```python
from build123d import *

# Parameters (mm, degrees)
SKETCH_1_R          = 4.5
EXTRUDE_1_DEPTH     = 2
SKETCH_2_R          = 3.5
CUT_EXTRUDE_1_DEPTH = 2
SKETCH_3_R          = 1.5
CUT_EXTRUDE_2_DEPTH = 7.670832032


with BuildPart() as part:
    # 草图1 → 凸台-拉伸1 (new, symmetric)
    with BuildSketch(Plane(origin=(0, 0, 0), x_dir=(1, 0, 0), z_dir=(0, 1, 0))):
        with Locations(Location((0, 0, 0), (0, 0, 270))):
            Circle(SKETCH_1_R)
    extrude(amount=EXTRUDE_1_DEPTH, both=True)

    # 草图2 → 切除-拉伸1 (cut)
    with BuildSketch(Plane(origin=(0, 2, 0), x_dir=(1, 0, 0), z_dir=(0, 1, 0))):
        with Locations(Location((0, 0, 0), (0, 0, 270))):
            Circle(SKETCH_2_R)
    extrude(amount=-CUT_EXTRUDE_1_DEPTH, mode=Mode.SUBTRACT)

    # 草图3 → 切除-拉伸2 (cut, through all)
    with BuildSketch(Plane(origin=(0, 0, 0), x_dir=(1, 0, 0), z_dir=(0, 1, 0))):
        with Locations(Location((0, 0, 0), (0, 0, 270))):
            Circle(SKETCH_3_R)
    extrude(amount=-CUT_EXTRUDE_2_DEPTH, mode=Mode.SUBTRACT)


solid = part.part
```
Work out the finished part from the listing and answer in its coordinate system (mm). Coordinates: 2 decimals unless noted, no trailing zeros. Loops run counter-clockwise (first coordinate to the right, second up) from the corner with the lowest first, then second, coordinate; pieces in that order, holes last. Notation, with made-up numbers: (1.25, 35.25) - (22.25, 35.25) arc R29 cw to (22.25, 70.25) - close; hole circle Ø3 at (44.5, 75). An arc over 180 degrees is marked (long way). Use a Markdown table: item, result.
Item 1: Find section A-A, the plane x = 0. Determine the outline of the cut face in (y, z), and give its area (3 significant figures).
Evaluation:
| item | result |
|---|---|
| outline | (-2, -4.5) - (2, -4.5) - (2, -3.5) - (0, -3.5) - (0, -1.5) - (-2, -1.5) - close; (-2, 1.5) - (0, 1.5) - (0, 3.5) - (2, 3.5) - (2, 4.5) - (-2, 4.5) - close |
| area | 16.0 mm2 |
Item 2: Find section C-C, the plane x = 2. Determine the outline of the cut face in (y, z), and give its area (3 significant figures).
Evaluation:
| item | result |
|---|---|
| outline | (-2, -4.03) - (2, -4.03) - (2, -2.87) - (0, -2.87) - (0, 2.87) - (2, 2.87) - (2, 4.03) - (-2, 4.03) - close |
| area | 20.8 mm2 |
Item 3: Find section B-B, the plane z = 0. Determine the outline of the cut face in (x, y).
Evaluation:
| item | result |
|---|---|
| outline | (-4.5, -2) - (-1.5, -2) - (-1.5, 0) - (-3.5, 0) - (-3.5, 2) - (-4.5, 2) - close; (1.5, -2) - (4.5, -2) - (4.5, 2) - (3.5, 2) - (3.5, 0) - (1.5, 0) - close |
Item 4: Given pin 1 Ø1.5 at (x, y) = (-3, 0) entering from -Z; pin 2 Ø3.5 at (x, z) = (1.5, 0.5) entering from +Y; pin 3 Ø2.5 at (x, z) = (0, 0) entering from +Y; pin 4 Ø2 at (x, y) = (-2, 1) entering from -Z, each flat-ended and moving along its own axis, determine where each tip first touches the part or whether it passes through.
Evaluation:
| item | result |
|---|---|
| pin 1 | stops at z = -3.9 |
| pin 2 | stops at y = 0 |
| pin 3 | passes through |
| pin 4 | stops at z = -4.39 |
Item 5: Find section D-D, the plane y = -0.15. Determine the outline of the cut face in (x, z).
Evaluation:
| item | result |
|---|---|
| outline | circle Ø9 at (0, 0); hole circle Ø3 at (0, 0) |
Item 6: The mould has two halves that part along Z. Classify faces 1 (the cylindrical face through (1.352, 0.028, 4.292)), 2 (the flat face through (-4, 2, 0)), 3 (the flat face through (0, 0, 2)), 4 (the cylindrical face through (-3.417, 1.014, -0.759)): +Z half, -Z half, draft (parallel to the pull), parting line (faces both ways), or undercut.
Evaluation:
| item | result |
|---|---|
| face 1 | parting line |
| face 2 | draft |
| face 3 | undercut |
| face 4 | undercut |
Item 7: Consider probe 1 along X at (y, z) = (-0.85, 0); probe 2 along X at (y, z) = (1.1, 0); probe 3 along Z at (x, y) = (-0.25, 0.2). Determine where each line is inside the solid, lowest interval first. Write a range as from..to.
Evaluation:
| item | result |
|---|---|
| probe 1 | x = -4.5..-1.5, 1.5..4.5 |
| probe 2 | x = -4.5..-3.5, 3.5..4.5 |
| probe 3 | z = -4.49..-3.49, 3.49..4.49 |
